The drawing under review shows one solid part. Ordinate dimensions are in mm from its lowest x, y, z. A direction names the side the tool comes from. Give positions to 0.01 mm unless a question says otherwise; leave off trailing zeros. Order: outer loops, then holes, each group sorted by start corner. A loop starts at its lowest first (then second) coordinate and runs counter-clockwise, first axis right, second up. Notation, with made-up numbers: (-9.75, 41.5) -> (6.25, 41.5) arc R7 cw to (6.25, 52.5) -> close; hole circle Ø7 at (20.5, -13). An arc over 180 degrees is marked (long way). One line per item, written item: value.
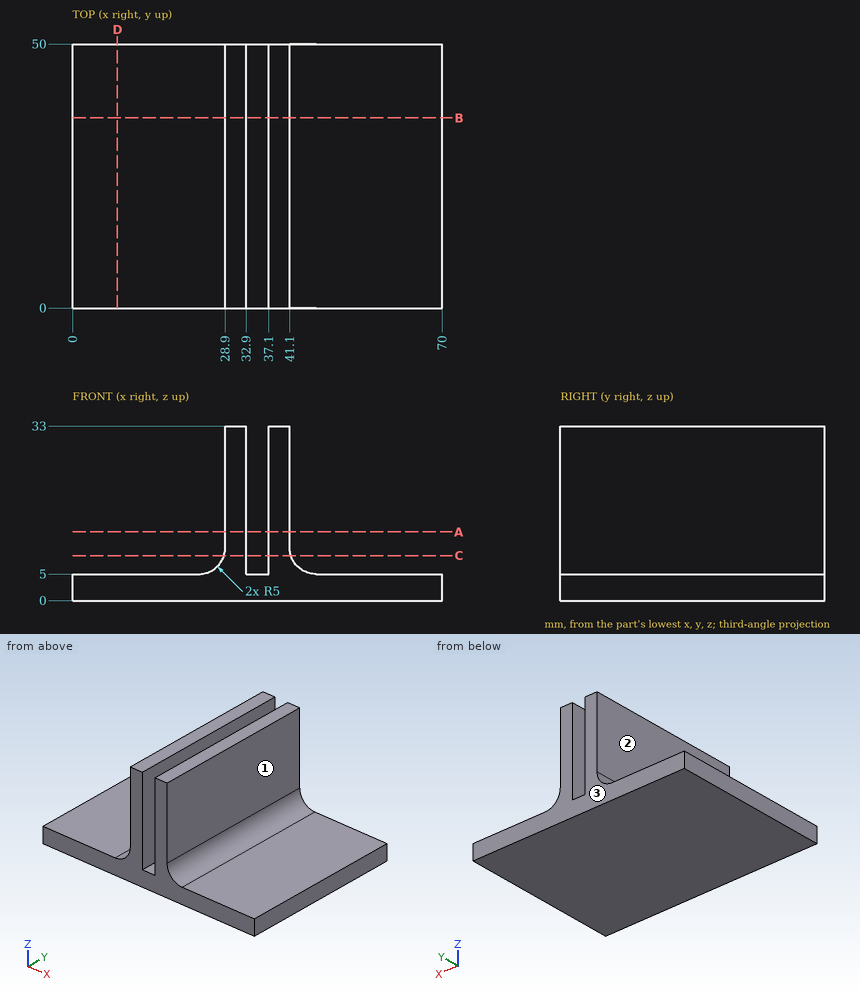
Item 1: Add section D-D on x = 8.5. Give the boundary of the cut face in (y, z).
Returned:
outline: (0, 0) -> (50, 0) -> (50, 5) -> (0, 5) -> close
Item 2: To check wall thickness, follow line 1 along X through (y, z) = (9.5, 13); line 2 along Z through (x, y) = (18.5, 42.5); line 3 along X through (y, z) = (24, 8.5). State the ranges of each line that lie inside material, in increasing order. Write a range as from..to.
Returned:
line 1: 28.9..32.9, 37.1..41.1
line 2: 0..5
line 3: 28.67..32.9, 37.1..41.33
Item 3: Clearance check with flat-ended pins moving along their axes: P1, Ø5, axis at x = 25.5, z = 8.5, coming from the +Y side; P2, Ø14, axis at y = 16, z = 19, coming from the +X side; P3, Ø7, axis at x = 15.5, y = 16.5, coming from the +Z side; P4, Ø12, axis at y = 22, z = 18, coming from the -X side. State where each tip first meets the part, or that it passes through.
Returned:
P1: through
P2: x = 41.1
P3: z = 5
P4: x = 28.9
Item 4: Machinability: for the marked faces 1, 2 and 3, which of the approach directions +Z, -Z, +X, -X, +Y, -Y give a long, thin tool a straight path to every point of the face, cutting with its end or side? Answer none if there is none.
Returned:
face 1: +Z, +X, +Y, -Y
face 2: +Z, -X, +Y, -Y
face 3: +Z, -Z, +X, -X, +Y
Item 5: Add section B-B on y = 36. Give the boundary of the cut face in (x, z).
Returned:
outline: (0, 0) -> (70, 0) -> (70, 5) -> (46.1, 5) arc R5 cw to (41.1, 10) -> (41.1, 33) -> (37.1, 33) -> (37.1, 5) -> (32.9, 5) -> (32.9, 33) -> (28.9, 33) -> (28.9, 10) arc R5 cw to (23.9, 5) -> (0, 5) -> close
Item 6: Add section C-C on z = 8.5. Give the boundary of the cut face in (x, y).
Returned:
outline: (28.67, 0) -> (32.9, 0) -> (32.9, 50) -> (28.67, 50) -> close; (37.1, 0) -> (41.33, 0) -> (41.33, 50) -> (37.1, 50) -> close
Item 7: Add section A-A on z = 13. Give the boundary of the cut face in (x, y).
Returned:
outline: (28.9, 0) -> (32.9, 0) -> (32.9, 50) -> (28.9, 50) -> close; (37.1, 0) -> (41.1, 0) -> (41.1, 50) -> (37.1, 50) -> close
